Autodesk Inventor part; units mm, degrees
ref_plane "Start plane" through (0, 0, -17.5) normal (0, 0, 1) x (1, 0, 0)
ref_plane "End plane" through (0, 0, 517.5) normal (0, 0, 1) x (1, 0, 0)
ref_plane "Work Plane4" through (17.5, 0, -17.5) normal (0, 0, -1) x (-1, 0, 0)
ref_plane "Start plane" through (0, 0, -17.5) normal (0, 0, 1) x (1, 0, 0)
ref_plane "End plane" through (0, 0, 517.5) normal (0, 0, 1) x (1, 0, 0)
sketch "Sketch" plane through (0, 0, 0) normal (0, 0, 1) x (1, 0, 0)
  line L0 (-17.5, -14.3) -> (-17.5, 14.3)
  line L1 (-14.3, 17.5) -> (14.3, 17.5)
  line L2 (17.5, 14.3) -> (17.5, -14.3)
  line L3 (14.3, -17.5) -> (-14.3, -17.5)
  arc A0 (-17.5, -14.3) -> (-14.3, -17.5) centre (-14.3, -14.3) ccw
  arc A1 (-14.3, 17.5) -> (-17.5, 14.3) centre (-14.3, 14.3) ccw
  arc A2 (17.5, 14.3) -> (14.3, 17.5) centre (14.3, 14.3) ccw
  arc A3 (14.3, -17.5) -> (17.5, -14.3) centre (14.3, -14.3) ccw
  arc A4 (-14.3, 15.9) -> (-15.9, 14.3) centre (-14.3, 14.3) ccw
  line L4 (-14.3, 15.9) -> (14.3, 15.9)
  arc A5 (15.9, 14.3) -> (14.3, 15.9) centre (14.3, 14.3) ccw
  line L5 (15.9, 14.3) -> (15.9, -14.3)
  arc A6 (14.3, -15.9) -> (15.9, -14.3) centre (14.3, -14.3) ccw
  line L6 (14.3, -15.9) -> (-14.3, -15.9)
  arc A7 (-15.9, -14.3) -> (-14.3, -15.9) centre (-14.3, -14.3) ccw
  line L7 (-15.9, -14.3) -> (-15.9, 14.3)
  line L8 (0, 25.4278) -> (0, -25.4278) construction
  line L9 (-25.4278, 0) -> (25.4278, 0) construction
  dimension "d7" = 3.2
  dimension "d10" = 35
  dimension "d11" = 35
  dimension "d12" = 1.6
  dimension "d15" = 17.5
  dimension "d16" = 17.5
extrude "Body" add sketch "Sketch" along normal up to surface (535 mm away) from surface at -17.5
sketch "Sketch3" plane through (0, 0, 0) normal (0, 0, 1) x (1, 0, 0)
  line L0 (0, 0) -> (10, 0)
ref_plane "Work Plane3" through (0, 0, 0) normal (0, -1, 0) x (1, 0, 0)
sketch "Sketch4" plane through (0, 0, 0) normal (0, -1, 0) x (1, 0, 0)
  line L0 (-2, -17.5) -> (12, -17.5)
  line L1 (-2, 517.5) -> (12, 517.5)
  dimension "d18" = 535
ref_plane "Work Plane4" through (17.5, 0, -17.5) normal (0, 0, -1) x (-1, 0, 0)
split "Split1" plane through (17.5, 0, -17.5) removes the side toward (0, 0, -1)
ref_plane "Work Plane5" through (0, 17.5, 517.5) normal (0, -0.7071, 0.7071) x (1, 0, 0)
split "Split2" plane through (0, 17.5, 517.5) removes the side toward (0, -0.7071, 0.7071)
ref_plane "Work Plane15" through (0, 17.5, -17.5) normal (0, -0.7071, -0.7071) x (1, 0, 0)
split "Split6" plane through (0, 17.5, -17.5) removes the side toward (0, -0.7071, -0.7071)
equation "\"d7\" = G_IR"
equation "\"d10\" = G_H"
equation "\"d11\" = G_W"
equation "\"d12\" = G_T"
equation "\"d15\" = 0.5 * d10"
equation "\"d16\" = 0.5 * d11"
equation "\"d3\" = G_L"
equation "\"G_W\" = 35"
equation "\"G_H\" = 35"
equation "\"G_T\" = 1.6"
equation "\"G_IR\" = 3.2"
equation "\"G_L\" = 535"
equation "\"G_OFFSET_START\" = 17.5"
equation "\"G_OFFSET_END\" = 17.5"
equation "\"d13\" = -G_OFFSET_START"
equation "\"d14\" = G_OFFSET_END + B_L"
properties part number "AS 1163 - C350L0 35x35x1.6 SHS - 535" material "Steel, Mild"
Geometry: final body of the model. Coordinates: model frame, mm. A direction names the side the tool comes from. Coordinates: 2 decimals unless noted, no trailing zeros. Write each loop counter-clockwise with the first axis right and the second up, starting at its lowest first coordinate (ties: lowest second). Pieces come first, ordered by that corner, then holes. Notation, with made-up numbers: M 4.5,33.25 L 12.5,33.25 A6 cw 12.5,38.25 Z; hole C -3,6 d2. An arc over 180 degrees is marked long. Use CSV: the item, a comma, the result in double quotes. Start each with the question number.
1. First-contact query: P1, Ø3, axis at x = -13.5, y = 10, coming from the -Z side. Flat tip, straight axial feed; report the tip coordinate or a pass-through.
2. Mould query, pull axis Y, two halves, no side actions, for faces 1 (the face through (0, -15.9, 247)), 2 (the face through (0, 17.5, 246)), 3 (the face through (-17.5, 0, 246)), 4 (the face through (17, -1, 499)). Classes: pulls with the +Y half, pulls with the -Y half, needs draft (parallel to the pull), parting line crosses it, or undercut.
3. Cut plane B-B on x = 1.5. Return the cut outline in (y, z).
4. Reachability of faces 5 (the face through (17.5, 0, 246)), 6 (the face through (-15.9, 0, 246)) from +Z, -Z, +X, -X, +Y, -Y: full face, straight path, thin tool, end or side. Return the list, or none.
5. Cut plane C-C on z = 235.5. Return the cut outline in (x, y), plus the area to 3 significant figures.
6. Ray query, probe 1 along Y at (x, z) = (1, 249); probe 2 along Z at (x, y) = (-8, 16). Return the intervals inside material, ascending.
7. Cut plane A-A on y = -1.5. Return the cut outline in (x, z).
Entries:
1,P1,"through"
2,face 1,"undercut"
2,face 2,"pulls with the +Y half"
2,face 3,"needs draft"
2,face 4,"pulls with the -Y half"
3,outline,"M -17.5,17.5 L -15.9,15.9 L -15.9,484.1 L -17.5,482.5 Z; M 15.9,-15.9 L 17.5,-17.5 L 17.5,517.5 L 15.9,515.9 Z"
4,face 5,"+Z, -Z, +X, +Y, -Y"
4,face 6,"+Z, -Z"
5,outline,"M -17.5,-14.3 A3.2 ccw -14.3,-17.5 L 14.3,-17.5 A3.2 ccw 17.5,-14.3 L 17.5,14.3 A3.2 ccw 14.3,17.5 L -14.3,17.5 A3.2 ccw -17.5,14.3 Z; hole M -15.9,-14.3 A1.6 ccw -14.3,-15.9 L 14.3,-15.9 A1.6 ccw 15.9,-14.3 L 15.9,14.3 A1.6 ccw 14.3,15.9 L -14.3,15.9 A1.6 ccw -15.9,14.3 Z"
5,area,"207 mm²"
6,probe 1,"-17.5 to -15.9, 15.9 to 17.5"
6,probe 2,"-16 to 516"
7,outline,"M -17.5,1.5 L -15.9,1.5 L -15.9,498.5 L -17.5,498.5 Z; M 15.9,1.5 L 17.5,1.5 L 17.5,498.5 L 15.9,498.5 Z"
